Verification items for this drawing (mm, ordinates from the low corner). A direction names the side the tool comes from. Give positions to 0.01 mm unless a question says otherwise; leave off trailing zeros. Write each loop counter-clockwise with the first axis right and the second up, starting at its lowest first coordinate (ties: lowest second). Pieces come first, ordered by that corner, then holes. Notation, with made-up numbers: M -34.5,44 L 19.5,44 A22 ccw 19.5,76 Z; hole C 86,37.5 d5. An arc over 180 degrees is marked long. Write each question's results on one line, items separated by ' | '.
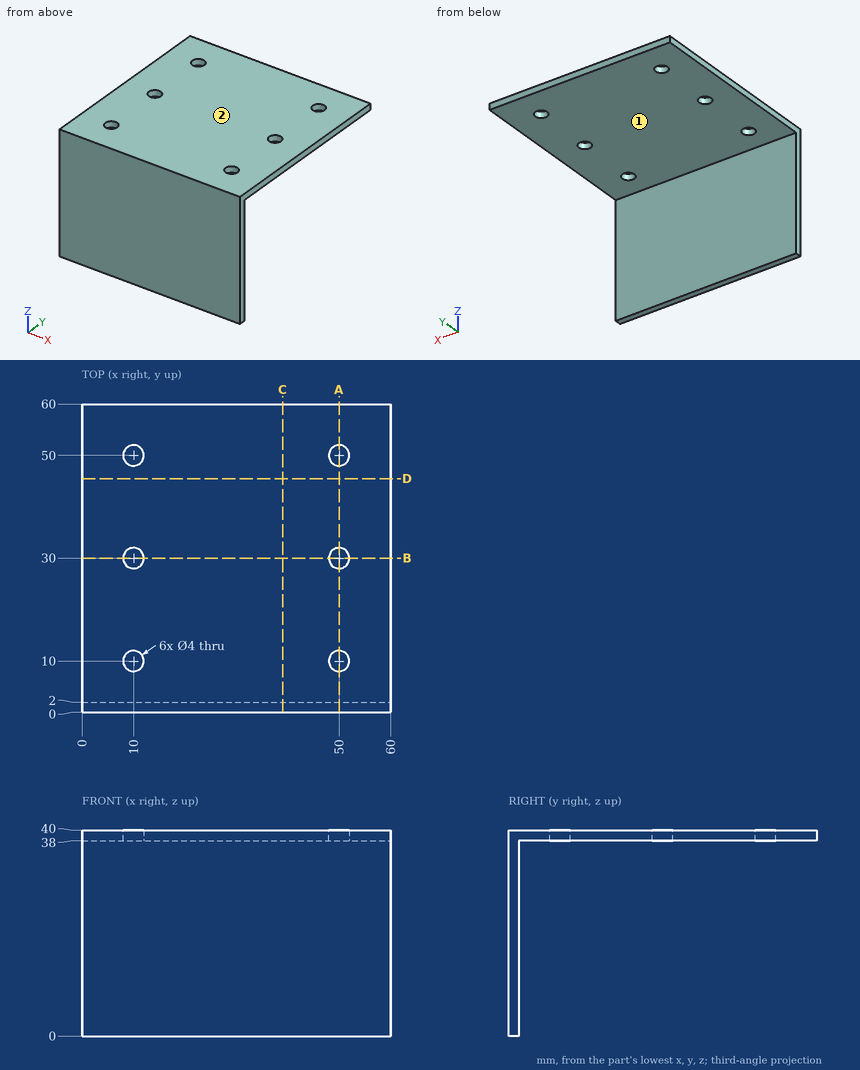
Q1. Section check A-A (x = 50). Enter the section's corners in (y, z), then the cut area to 3 significant figures.
Answer key:
outline: M 0,0 L 2,0 L 2,38 L 8,38 L 8,40 L 0,40 Z; M 12,38 L 28,38 L 28,40 L 12,40 Z; M 32,38 L 48,38 L 48,40 L 32,40 Z; M 52,38 L 60,38 L 60,40 L 52,40 Z | area: 172 mm2
Q2. Material ranges on probe 1 along Y at (x, z) = (10, 39); probe 2 along Z at (x, y) = (39, 40); probe 3 along Y at (x, z) = (20.5, 9), recorded low to high. Write a range as [from, to].
Answer key:
probe 1: y = [0, 8], [12, 28], [32, 48], [52, 60] | probe 2: z = [38, 40] | probe 3: y = [0, 2]
Q3. Depth check by flat-ended pin: P1, Ø8, axis at x = 34.5, z = 7.5, coming from the +Y side. Enter the tip coordinate at first touch or a pass-through.
Answer key:
P1: stops at y = 2
Q4. Access from +Z, -Z, +X, -X, +Y, -Y to the whole of each face (thin tool, end or side, straight path). Record for the marked faces 1 and 2.
Answer key:
face 1: -Z, +X, -X, +Y | face 2: +Z, +X, -X, +Y, -Y
Q5. Section check D-D (y = 45.5). Enter the section's corners in (x, z), then the cut area to 3 significant figures.
Answer key:
outline: M 0,38 L 60,38 L 60,40 L 0,40 Z | area: 120 mm2
Q6. Section check C-C (x = 39). Enter the section's corners in (y, z), then the cut area to 3 significant figures.
Answer key:
outline: M 0,0 L 2,0 L 2,38 L 60,38 L 60,40 L 0,40 Z | area: 196 mm2
Q7. Section check B-B (y = 30). Enter the section's corners in (x, z), then the cut area to 3 significant figures.
Answer key:
outline: M 0,38 L 8,38 L 8,40 L 0,40 Z; M 12,38 L 48,38 L 48,40 L 12,40 Z; M 52,38 L 60,38 L 60,40 L 52,40 Z | area: 104 mm2
